```python
from build123d import *

# Parameters (mm, degrees)
F0_W     = 21.5
F0_H     = 29.7
F1_DEPTH = 32.4
F2_R     = 6
F3_DEPTH = 10.5


with BuildPart() as f1:
    # F0 (on Front) → F1 (new body)
    with BuildSketch(Plane.XZ):
        Rectangle(F0_W, F0_H)
    extrude(amount=-F1_DEPTH)

    # F2 (on face) → F3 (join)
    with BuildSketch(Plane.XZ):
        Circle(F2_R)
    extrude(amount=F3_DEPTH)


solid = f1.part
```
Model file for the job. Use its own axes, mm. A direction names the side the tool comes from. Coordinates: 2 decimals unless noted, no trailing zeros. Order: outer loops, then holes, each group sorted by start corner. A loop starts at its lowest first (then second) coordinate and runs counter-clockwise, first axis right, second up. Notation, with made-up numbers: (40, -15.5) -> (83, -15.5) arc R6 cw to (83, -8.5) -> close; hole circle Ø5 at (0.5, 75.5). An arc over 180 degrees is marked (long way). Return JSON: item names as keys, results as strings.
Item 1: 3-axis set-ups, long thin cutter, end or side, ignore diameter. For faces 1 (the face through (0, 32.4, 0)), 2 (the face through (-6, -5, 0)): which of +Z, -Z, +X, -X, +Y, -Y reach the whole face in a straight line?
Model answer:
{"face 1": "+Z, -Z, +X, -X, +Y", "face 2": "-Y"}
Item 2: Slice it at A-A (x = 0). Write the cut outline in (y, z), then the cut area to 3 significant figures.
Model answer:
{"outline": "(-10.5, -6) -> (0, -6) -> (0, -14.85) -> (32.4, -14.85) -> (32.4, 14.85) -> (0, 14.85) -> (0, 6) -> (-10.5, 6) -> close", "area": "1,090 mm²"}
Item 3: Slice it at D-D (x = -7). Write the cut outline in (y, z).
Model answer:
{"outline": "(0, -14.85) -> (32.4, -14.85) -> (32.4, 14.85) -> (0, 14.85) -> close"}
Item 4: Slice it at C-C (z = -12). Write the cut outline in (x, y), then the cut area to 3 significant figures.
Model answer:
{"outline": "(-10.75, 0) -> (10.75, 0) -> (10.75, 32.4) -> (-10.75, 32.4) -> close", "area": "697 mm²"}
Item 5: Wall check: line 1 along Y through (x, z) = (0.25, 7.75); line 2 along X through (y, z) = (-5, 0.25); line 3 along Z through (x, y) = (-3, -3). Give the ranges that are in metal, low to high. Write a range as from..to.
Model answer:
{"line 1": "y = 0..32.4", "line 2": "x = -5.99..5.99", "line 3": "z = -5.2..5.2"}
Item 6: Pin check, flat tip, straight feed: P1, Ø6, axis at x = 6.5, z = -6.5, coming from the -Y side. Stop position of the tip, or through.
Model answer:
{"P1": "stops at y = 0"}
Item 7: Slice it at B-B (z = 0). Write the cut outline in (x, y).
Model answer:
{"outline": "(-10.75, 0) -> (-6, 0) -> (-6, -10.5) -> (6, -10.5) -> (6, 0) -> (10.75, 0) -> (10.75, 32.4) -> (-10.75, 32.4) -> close"}
